from build123d import *

# Parameters (mm, degrees)
EXTRUDE_1_DEPTH          = 140
FILLET_1_R               = 0.2
CUT_EXTRUDE_1_DEPTH      = 149.996644258
CUT_EXTRUDE_1_DEPTH_BACK = 149.996644258
SKETCH_2_W               = 41.416635457
SKETCH_2_H               = 21.85529521


with BuildPart() as part:
    # 草图1 → 凸台-拉伸1 (new body)
    with BuildSketch(Plane(origin=(0, 0, 0), x_dir=(1, 0, 0), z_dir=(0, 1, 0))):
        with BuildLine():
            Line((-3.476396103, 2.84), (-3.476396103, 0))
            Line((-3.476396103, 0), (-2.1, 0))
            ThreePointArc((-2.1, 0), (-1.48492424, 1.48492424), (0, 2.1))
            Line((0, 2.1), (0, 3.476396103))
            Line((0, 3.476396103), (-2.84, 3.476396103))
            Line((-2.84, 3.476396103), (-5.923603897, 6.56))
            Line((-5.923603897, 6.56), (-5.923603897, 8.2))
            Line((-5.923603897, 8.2), (-3.1, 8.2))
            Line((-3.1, 8.2), (-4.9, 10))
            Line((-4.9, 10), (-10, 10))
            Line((-10, 10), (-10, 4.9))
            Line((-10, 4.9), (-8.2, 3.1))
            Line((-8.2, 3.1), (-8.2, 5.923603897))
            Line((-8.2, 5.923603897), (-6.56, 5.923603897))
            Line((-6.56, 5.923603897), (-3.476396103, 2.84))
        make_face()
        with BuildLine():
            Line((-2.1, 0), (-3.476396103, 0))
            Line((-3.476396103, 0), (-3.476396103, -2.84))
            Line((-3.476396103, -2.84), (-6.56, -5.923603897))
            Line((-6.56, -5.923603897), (-8.2, -5.923603897))
            Line((-8.2, -5.923603897), (-8.2, -3.1))
            Line((-8.2, -3.1), (-10, -4.9))
            Line((-10, -4.9), (-10, -10))
            Line((-10, -10), (-4.9, -10))
            Line((-4.9, -10), (-3.1, -8.2))
            Line((-3.1, -8.2), (-5.923603897, -8.2))
            Line((-5.923603897, -8.2), (-5.923603897, -6.56))
            Line((-5.923603897, -6.56), (-2.84, -3.476396103))
            Line((-2.84, -3.476396103), (0, -3.476396103))
            Line((0, -3.476396103), (0, -2.1))
            ThreePointArc((0, -2.1), (-1.48492424, -1.48492424), (-2.1, 0))
        make_face()
        with BuildLine():
            ThreePointArc((2.1, 0), (1.48492424, -1.48492424), (0, -2.1))
            Line((0, -2.1), (0, -3.476396103))
            Line((0, -3.476396103), (2.84, -3.476396103))
            Line((2.84, -3.476396103), (5.923603897, -6.56))
            Line((5.923603897, -6.56), (5.923603897, -8.2))
            Line((5.923603897, -8.2), (3.1, -8.2))
            Line((3.1, -8.2), (4.9, -10))
            Line((4.9, -10), (15.1, -10))
            Line((15.1, -10), (16.9, -8.2))
            Line((16.9, -8.2), (14.076396103, -8.2))
            Line((14.076396103, -8.2), (14.076396103, -6.56))
            Line((14.076396103, -6.56), (17.16, -3.476396103))
            Line((17.16, -3.476396103), (20, -3.476396103))
            Line((20, -3.476396103), (20, -2.1))
            ThreePointArc((20, -2.1), (18.51507576, -1.48492424), (17.9, 0))
            Line((17.9, 0), (16.523603897, 0))
            Line((16.523603897, 0), (16.523603897, -2.84))
            Line((16.523603897, -2.84), (13.44, -5.923603897))
            Line((13.44, -5.923603897), (11.163603897, -8.2))
            Line((11.163603897, -8.2), (8.836396103, -8.2))
            Line((8.836396103, -8.2), (6.56, -5.923603897))
            Line((6.56, -5.923603897), (3.476396103, -2.84))
            Line((3.476396103, -2.84), (3.476396103, 0))
            Line((3.476396103, 0), (2.1, 0))
        make_face()
        with BuildLine():
            Line((0, 3.476396103), (0, 2.1))
            ThreePointArc((0, 2.1), (1.48492424, 1.48492424), (2.1, 0))
            Line((2.1, 0), (3.476396103, 0))
            Line((3.476396103, 0), (3.476396103, 2.84))
            Line((3.476396103, 2.84), (6.56, 5.923603897))
            Line((6.56, 5.923603897), (8.836396103, 8.2))
            Line((8.836396103, 8.2), (11.163603897, 8.2))
            Line((11.163603897, 8.2), (13.44, 5.923603897))
            Line((13.44, 5.923603897), (16.523603897, 2.84))
            Line((16.523603897, 2.84), (16.523603897, 0))
            Line((16.523603897, 0), (17.9, 0))
            ThreePointArc((17.9, 0), (18.51507576, 1.48492424), (20, 2.1))
            Line((20, 2.1), (20, 3.476396103))
            Line((20, 3.476396103), (17.16, 3.476396103))
            Line((17.16, 3.476396103), (14.076396103, 6.56))
            Line((14.076396103, 6.56), (14.076396103, 8.2))
            Line((14.076396103, 8.2), (16.9, 8.2))
            Line((16.9, 8.2), (15.1, 10))
            Line((15.1, 10), (4.9, 10))
            Line((4.9, 10), (3.1, 8.2))
            Line((3.1, 8.2), (5.923603897, 8.2))
            Line((5.923603897, 8.2), (5.923603897, 6.56))
            Line((5.923603897, 6.56), (2.84, 3.476396103))
            Line((2.84, 3.476396103), (0, 3.476396103))
        make_face()
        with BuildLine():
            Line((20, 3.476396103), (20, 2.1))
            ThreePointArc((20, 2.1), (21.48492424, 1.48492424), (22.1, 0))
            Line((22.1, 0), (23.476396103, 0))
            Line((23.476396103, 0), (23.476396103, 2.84))
            Line((23.476396103, 2.84), (26.56, 5.923603897))
            Line((26.56, 5.923603897), (28.836396103, 8.2))
            Line((28.836396103, 8.2), (31.163603897, 8.2))
            Line((31.163603897, 8.2), (33.44, 5.923603897))
            Line((33.44, 5.923603897), (36.523603897, 2.84))
            Line((36.523603897, 2.84), (36.523603897, 0))
            Line((36.523603897, 0), (37.9, 0))
            ThreePointArc((37.9, 0), (40, 2.1), (42.1, 0))
            Line((42.1, 0), (43.476396103, 0))
            Line((43.476396103, 0), (43.476396103, 2.84))
            Line((43.476396103, 2.84), (46.56, 5.923603897))
            Line((46.56, 5.923603897), (48.2, 5.923603897))
            Line((48.2, 5.923603897), (48.2, 3.1))
            Line((48.2, 3.1), (50, 4.9))
            Line((50, 4.9), (50, 10))
            Line((50, 10), (44.9, 10))
            Line((44.9, 10), (43.1, 8.2))
            Line((43.1, 8.2), (45.923603897, 8.2))
            Line((45.923603897, 8.2), (45.923603897, 6.56))
            Line((45.923603897, 6.56), (42.84, 3.476396103))
            Line((42.84, 3.476396103), (37.16, 3.476396103))
            Line((37.16, 3.476396103), (34.076396103, 6.56))
            Line((34.076396103, 6.56), (34.076396103, 8.2))
            Line((34.076396103, 8.2), (36.9, 8.2))
            Line((36.9, 8.2), (35.1, 10))
            Line((35.1, 10), (24.9, 10))
            Line((24.9, 10), (23.1, 8.2))
            Line((23.1, 8.2), (25.923603897, 8.2))
            Line((25.923603897, 8.2), (25.923603897, 6.56))
            Line((25.923603897, 6.56), (22.84, 3.476396103))
            Line((22.84, 3.476396103), (20, 3.476396103))
        make_face()
        with BuildLine():
            ThreePointArc((22.1, 0), (21.48492424, -1.48492424), (20, -2.1))
            Line((20, -2.1), (20, -3.476396103))
            Line((20, -3.476396103), (22.84, -3.476396103))
            Line((22.84, -3.476396103), (25.923603897, -6.56))
            Line((25.923603897, -6.56), (25.923603897, -8.2))
            Line((25.923603897, -8.2), (23.1, -8.2))
            Line((23.1, -8.2), (24.9, -10))
            Line((24.9, -10), (35.1, -10))
            Line((35.1, -10), (36.9, -8.2))
            Line((36.9, -8.2), (34.076396103, -8.2))
            Line((34.076396103, -8.2), (34.076396103, -6.56))
            Line((34.076396103, -6.56), (37.16, -3.476396103))
            Line((37.16, -3.476396103), (42.84, -3.476396103))
            Line((42.84, -3.476396103), (45.923603897, -6.56))
            Line((45.923603897, -6.56), (45.923603897, -8.2))
            Line((45.923603897, -8.2), (43.1, -8.2))
            Line((43.1, -8.2), (44.9, -10))
            Line((44.9, -10), (50, -10))
            Line((50, -10), (50, -4.9))
            Line((50, -4.9), (48.2, -3.1))
            Line((48.2, -3.1), (48.2, -5.923603897))
            Line((48.2, -5.923603897), (46.56, -5.923603897))
            Line((46.56, -5.923603897), (43.476396103, -2.84))
            Line((43.476396103, -2.84), (43.476396103, 0))
            Line((43.476396103, 0), (42.1, 0))
            ThreePointArc((42.1, 0), (40, -2.1), (37.9, 0))
            Line((37.9, 0), (36.523603897, 0))
            Line((36.523603897, 0), (36.523603897, -2.84))
            Line((36.523603897, -2.84), (33.44, -5.923603897))
            Line((33.44, -5.923603897), (31.163603897, -8.2))
            Line((31.163603897, -8.2), (28.836396103, -8.2))
            Line((28.836396103, -8.2), (26.56, -5.923603897))
            Line((26.56, -5.923603897), (23.476396103, -2.84))
            Line((23.476396103, -2.84), (23.476396103, 0))
            Line((23.476396103, 0), (22.1, 0))
        make_face()
    extrude(amount=EXTRUDE_1_DEPTH)

    # 圆角1
    fillet_1_edges = [part.edges().sort_by_distance(p)[0] for p in [
        (8.836396103, 70, 8.2),
        (11.163603897, 70, 8.2),
        (16.523603897, 70, 2.84),
        (16.523603897, 70, -2.84),
        (11.163603897, 70, -8.2),
        (8.836396103, 70, -8.2),
        (3.476396103, 70, -2.84),
        (3.476396103, 70, 2.84),
        (28.836396103, 70, 8.2),
        (31.163603897, 70, 8.2),
        (36.523603897, 70, 2.84),
        (36.523603897, 70, -2.84),
        (31.163603897, 70, -8.2),
        (28.836396103, 70, -8.2),
        (23.476396103, 70, -2.84),
        (23.476396103, 70, 2.84),
        (46.56, 70, 5.923603897),
        (48.2, 70, 5.923603897),
        (48.2, 70, 3.1),
        (50, 70, 4.9),
        (50, 70, 10),
        (44.9, 70, 10),
        (43.1, 70, 8.2),
        (45.923603897, 70, 8.2),
        (45.923603897, 70, 6.56),
        (42.84, 70, 3.476396103),
        (37.16, 70, 3.476396103),
        (34.076396103, 70, 6.56),
        (34.076396103, 70, 8.2),
        (36.9, 70, 8.2),
        (35.1, 70, 10),
        (24.9, 70, 10),
        (23.1, 70, 8.2),
        (25.923603897, 70, 8.2),
        (25.923603897, 70, 6.56),
        (22.84, 70, 3.476396103),
        (17.16, 70, 3.476396103),
        (14.076396103, 70, 6.56),
        (14.076396103, 70, 8.2),
        (16.9, 70, 8.2),
        (15.1, 70, 10),
        (4.9, 70, 10),
        (3.1, 70, 8.2),
        (5.923603897, 70, 8.2),
        (5.923603897, 70, 6.56),
        (2.84, 70, 3.476396103),
        (-2.84, 70, 3.476396103),
        (-5.923603897, 70, 6.56),
        (-5.923603897, 70, 8.2),
        (-3.1, 70, 8.2),
        (-4.9, 70, 10),
        (-10, 70, 10),
        (-10, 70, 4.9),
        (-8.2, 70, 3.1),
        (-8.2, 70, 5.923603897),
        (-6.56, 70, 5.923603897),
        (-3.476396103, 70, 2.84),
        (-3.476396103, 70, -2.84),
        (-6.56, 70, -5.923603897),
        (-8.2, 70, -5.923603897),
        (-8.2, 70, -3.1),
        (-10, 70, -4.9),
        (-10, 70, -10),
        (-4.9, 70, -10),
        (-3.1, 70, -8.2),
        (-5.923603897, 70, -8.2),
        (-5.923603897, 70, -6.56),
        (-2.84, 70, -3.476396103),
        (2.84, 70, -3.476396103),
        (5.923603897, 70, -6.56),
        (5.923603897, 70, -8.2),
        (3.1, 70, -8.2),
        (4.9, 70, -10),
        (15.1, 70, -10),
        (16.9, 70, -8.2),
        (14.076396103, 70, -8.2),
        (14.076396103, 70, -6.56),
        (17.16, 70, -3.476396103),
        (22.84, 70, -3.476396103),
        (25.923603897, 70, -6.56),
        (25.923603897, 70, -8.2),
        (23.1, 70, -8.2),
        (24.9, 70, -10),
        (35.1, 70, -10),
        (36.9, 70, -8.2),
        (34.076396103, 70, -8.2),
        (34.076396103, 70, -6.56),
        (37.16, 70, -3.476396103),
        (42.84, 70, -3.476396103),
        (45.923603897, 70, -6.56),
        (45.923603897, 70, -8.2),
        (43.1, 70, -8.2),
        (44.9, 70, -10),
        (50, 70, -10),
        (50, 70, -4.9),
        (48.2, 70, -3.1),
        (48.2, 70, -5.923603897),
        (46.56, 70, -5.923603897),
        (43.476396103, 70, -2.84),
        (43.476396103, 70, 2.84),
    ]]
    fillet(fillet_1_edges, radius=FILLET_1_R)

    # 草图2 → 切除-拉伸1 (cut, two sides: drawn at the far end of the back side and taken through both)
    with BuildSketch(Plane.XZ.offset(-CUT_EXTRUDE_1_DEPTH_BACK)):
        with Locations((30.708317729, -0.927647605)):
            Rectangle(SKETCH_2_W, SKETCH_2_H)
    extrude(amount=CUT_EXTRUDE_1_DEPTH + CUT_EXTRUDE_1_DEPTH_BACK, mode=Mode.SUBTRACT)


solid = part.part
Geometry check sheet. Reference: the model listing, model coordinates, mm. A direction names the side the tool comes from. Give positions to 0.01 mm unless a question says otherwise; leave off trailing zeros. Answer as a JSON object with one key per item and string values. Group by question number.
Item 1: Material ranges on L1, parallel to X at y = 35.5, z = 4.75; L2, parallel to Z at x = -4.75, y = 124.5; L3, parallel to Z at x = -7.25, y = 41, recorded low to high.
Item 2: Access from +Z, -Z, +X, -X, +Y, -Y to the whole of each face (thin tool, end or side, straight path). Record for faces 5 (the flat face through (-3.476, 69, 0)), 6 (the flat face through (3.476, 69, 0)), 7 (the flat face through (8, 69, -10)), 8 (the flat face through (-4.403, 69.02, 5.039)), 9 (the flat face through (0, 69, 3.476)).
Item 3: Mould release check, pull along Z, two halves, no side actions. Record for faces 1 (the flat face through (0, 69, -3.476)), 2 (the flat face through (-4.361, 69.02, -4.997)), 3 (the flat face through (-7, 69, 10)), 4 (the flat face through (-10, 69, 7)): pulls with the +Z half, pulls with the -Z half, needs draft (parallel to the pull), parting line crosses it, or undercut.
Item 4: Gauge pin test, flat ends, axial feed: pin 1 (0.6 mm diameter, centred on y = 103.5, z = 5, fed in from +X); pin 2 (2 mm diameter, centred on x = 2.5, y = 44, fed in from +Z); pin 3 (8 mm diameter, centred on x = -2.5, z = -1, fed in from -Y); pin 4 (1.1 mm diameter, centred on y = 46.5, z = -5, fed in from +X). Record the tip position at first contact, or that the pin passes through.
Findings below:
{
 "1": {"L1": "-9.85 to -8.2, -5.39 to -4.11, 4.11 to 5.39", "L2": "-9.85 to -8.2, -5.39 to -4.11, 4.11 to 5.39, 8.2 to 9.85", "L3": "-10 to -5.92, 5.92 to 10"},
 "2": {"face 5": "-X, +Y, -Y", "face 6": "+X, +Y, -Y", "face 7": "-Z, +X, -X, +Y, -Y", "face 8": "+Y, -Y", "face 9": "+Z, +Y, -Y"},
 "3": {"face 1": "pulls with the -Z half", "face 2": "undercut", "face 3": "pulls with the +Z half", "face 4": "needs draft"},
 "4": {"pin 1": "x = 5.94", "pin 2": "z = 8.6", "pin 3": "y = 0", "pin 4": "x = 6.19"}
}
